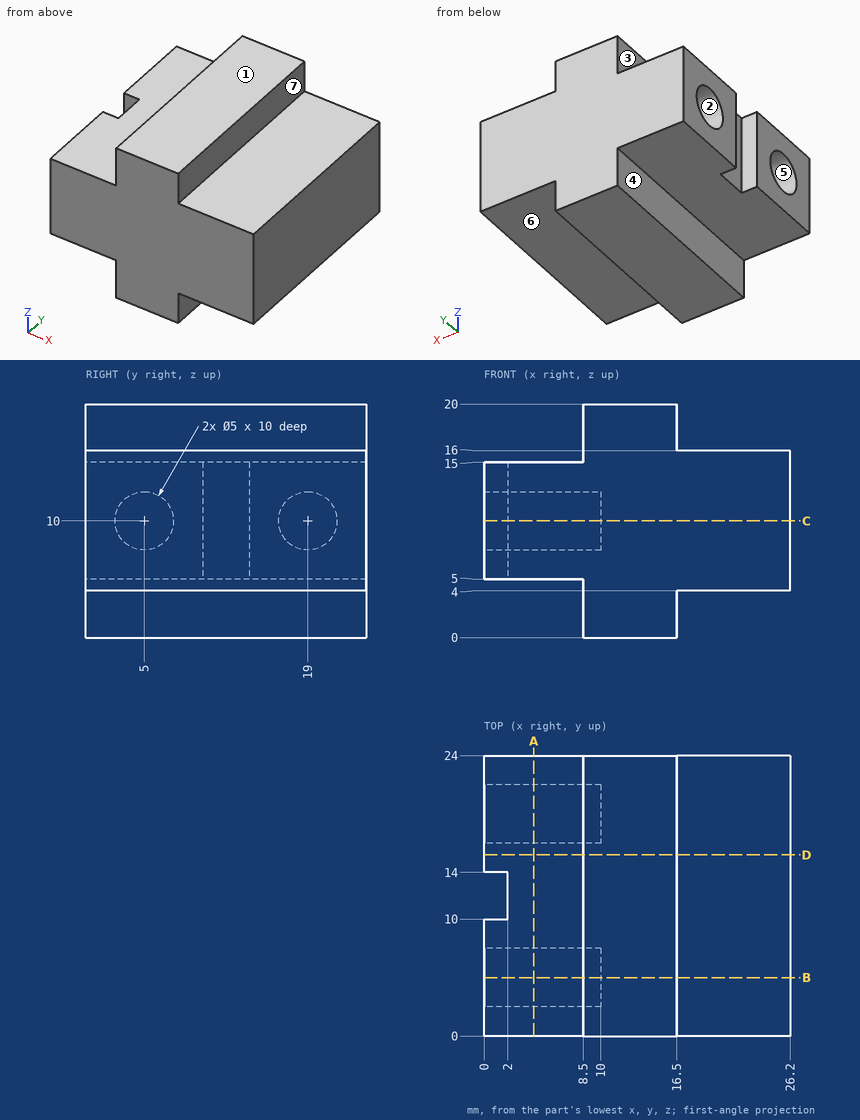
Drawing for the job (mm, zero at the part's lowest x, y, z). A direction names the side the tool comes from. Coordinates: 2 decimals unless noted, no trailing zeros. Order: outer loops, then holes, each group sorted by start corner. A loop starts at its lowest first (then second) coordinate and runs counter-clockwise, first axis right, second up. Notation, with made-up numbers: (41.25, -20.5) - (100.25, -20.5) arc R11 ccw to (100.25, 0.5) - close; hole circle Ø3 at (40.5, -14). An arc over 180 degrees is marked (long way). Use a Markdown table: item, result. Add a question column.
(1) Flat gauge pins, fed straight in: pin 1 (2.5 mm diameter, centred on y = 6, z = 10.5, fed in from -X); pin 2 (2 mm diameter, centred on y = 11.5, z = 2.5, fed in from +X); pin 3 (5 mm diameter, centred on x = 21, y = 8, fed in from +Z). Where does each tip first touch, or does it go through?
(2) Drill centre lines: line 1 along Y through (x, z) = (4.75, 10); line 2 along Y through (x, z) = (3.25, 8.75); line 3 along Z through (x, y) = (5.25, 16.25). Where is each one in solid material? Low to high. Write a range as [from, to].
(3) Which spindle directions (+Z, -Z, +X, -X, +Y, -Y) get a long thin tool onto all of the face, cutting with end or side? Do the marked faces 4, 5, 6 and 7. Say none if no direction does.
(4) Pull direction Z, two halves, no side cores. Call the marked faces 1, 2 and 3: +Z half, -Z half, draft (parallel to the pull), parting line (faces both ways), or undercut.
(5) Saw through at D-D (y = 15.5). Give the cut face in (x, z), then the cut area to 3 significant figures.
(6) Saw through at C-C (z = 10). Give the cut face in (x, y), then the cut area to 3 significant figures.
(7) Saw through at B-B (y = 5). Give the cut face in (x, z).
(8) Saw through at A-A (x = 4.25). Give the cut face in (y, z).
Solved:
| question | item | result |
|---|---|---|
| 1 | pin 1 | stops at x = 10 |
| 1 | pin 2 | stops at x = 16.5 |
| 1 | pin 3 | stops at z = 16 |
| 2 | line 1 | y = [0, 2.5], [7.5, 16.5], [21.5, 24] |
| 2 | line 2 | y = [0, 2.83], [7.17, 16.83], [21.17, 24] |
| 2 | line 3 | z = [5, 15] |
| 3 | face 4 | -Z, -X, +Y, -Y |
| 3 | face 5 | -X |
| 3 | face 6 | -Z, +X, +Y, -Y |
| 3 | face 7 | +Z, +X, +Y, -Y |
| 4 | face 1 | +Z half |
| 4 | face 2 | undercut |
| 4 | face 3 | draft |
| 5 | outline | (0, 5) - (8.5, 5) - (8.5, 0) - (16.5, 0) - (16.5, 4) - (26.2, 4) - (26.2, 16) - (16.5, 16) - (16.5, 20) - (8.5, 20) - (8.5, 15) - (0, 15) - close |
| 5 | area | 361 mm² |
| 6 | outline | (0, 0) - (26.2, 0) - (26.2, 24) - (0, 24) - (0, 21.5) - (10, 21.5) - (10, 16.5) - (0, 16.5) - (0, 14) - (2, 14) - (2, 10) - (0, 10) - (0, 7.5) - (10, 7.5) - (10, 2.5) - (0, 2.5) - close |
| 6 | area | 521 mm² |
| 7 | outline | (0, 5) - (8.5, 5) - (8.5, 0) - (16.5, 0) - (16.5, 4) - (26.2, 4) - (26.2, 16) - (16.5, 16) - (16.5, 20) - (8.5, 20) - (8.5, 15) - (0, 15) - (0, 12.5) - (10, 12.5) - (10, 7.5) - (0, 7.5) - close |
| 8 | outline | (0, 5) - (24, 5) - (24, 15) - (0, 15) - close; hole circle Ø5 at (5, 10); hole circle Ø5 at (19, 10) |
